Read the model definition and answer for the solid it produces. Units are mm, in the model's axes. A direction names the side the tool comes from. Round coordinates to 2 decimals unless told otherwise and drop trailing zeros. Order: outer loops, then holes, each group sorted by start corner. A loop starts at its lowest first (then second) coordinate and runs counter-clockwise, first axis right, second up.
from build123d import *

# Parameters (mm, degrees)
BENCH_FOOTPRINT_140X120_PROFILE_W       = 140
BENCH_FOOTPRINT_140X120_PROFILE_H       = 120
BENCH_FOOTPRINT_140X120_DEPTH           = 5
BACKBONE_START                          = -20
BACKBONE_PROFILE_W                      = 14
BACKBONE_PROFILE_H                      = 63
BACKBONE_DEPTH                          = 40
REMOVABLE_SERVO_MOUNT_M3_START          = -40
REMOVABLE_SERVO_MOUNT_M3_PROFILE_R      = 1.6
REMOVABLE_SERVO_MOUNT_M3_DEPTH          = 155.560027933
BEARING_BRIDGE_START                    = 39
BEARING_BRIDGE_PROFILE_W                = 53
BEARING_BRIDGE_PROFILE_H                = 40
BEARING_BRIDGE_DEPTH                    = 4
BRIDGE_HORN_CLEARANCE_START             = 38
BRIDGE_HORN_CLEARANCE_PROFILE_R         = 14
BRIDGE_HORN_CLEARANCE_DEPTH             = 77.560027933
DRIVE_COLLAR_CHAMBER_START              = 43
DRIVE_COLLAR_CHAMBER_PROFILE_R          = 18
DRIVE_COLLAR_CHAMBER_PROFILE_R_2        = 14
DRIVE_COLLAR_CHAMBER_DEPTH              = 5
BEARING_TOWER_START                     = 48
BEARING_TOWER_PROFILE_R                 = 18
BEARING_TOWER_PROFILE_R_2               = 11.1
BEARING_TOWER_DEPTH                     = 23
BEARING_SEPARATION_SHOULDER_START       = 55
BEARING_SEPARATION_SHOULDER_PROFILE_R   = 11.1
BEARING_SEPARATION_SHOULDER_PROFILE_R_2 = 9
BEARING_SEPARATION_SHOULDER_DEPTH       = 8
BENCH_CLAMP_HOLES_START                 = -1
BENCH_CLAMP_HOLES_PROFILE_R             = 2.75
BENCH_CLAMP_HOLES_DEPTH                 = 118.365802537
YAW_CROSSBOLT_ACCESS_START              = -40
YAW_CROSSBOLT_ACCESS_PROFILE_R          = 2.5
YAW_CROSSBOLT_ACCESS_DEPTH              = 157.365802537


with BuildPart() as part:
    # Bench_footprint_140x120_profile → Bench_footprint_140x120 (new body)
    with BuildSketch(Plane(origin=(0, 0, 0), x_dir=(1, 0, 0), z_dir=(0, 1, 0))):
        Rectangle(BENCH_FOOTPRINT_140X120_PROFILE_W, BENCH_FOOTPRINT_140X120_PROFILE_H)
    extrude(amount=BENCH_FOOTPRINT_140X120_DEPTH)

    # Backbone_profile → Backbone (add)
    with BuildSketch(Plane.XY.offset(BACKBONE_START)):
        with Locations((-28, 36.5)):
            Rectangle(BACKBONE_PROFILE_W, BACKBONE_PROFILE_H)
    extrude(amount=BACKBONE_DEPTH)

    # Removable_servo_mount_M3_profile → Removable_servo_mount_M3 (cut, through all)
    with BuildSketch(Plane(origin=(0, 0, 0), x_dir=(0, 0, -1), z_dir=(1, 0, 0)).offset(REMOVABLE_SERVO_MOUNT_M3_START)):
        with Locations(Location((12, 28, 0), (0, 0, 180))):
            Circle(REMOVABLE_SERVO_MOUNT_M3_PROFILE_R)
        with Locations(Location((-12, 28, 0), (0, 0, 180))):
            Circle(REMOVABLE_SERVO_MOUNT_M3_PROFILE_R)
    extrude(amount=REMOVABLE_SERVO_MOUNT_M3_DEPTH, mode=Mode.SUBTRACT)

    # Bearing_bridge_profile → Bearing_bridge (add)
    with BuildSketch(Plane(origin=(0, 0, 0), x_dir=(1, 0, 0), z_dir=(0, 1, 0)).offset(BEARING_BRIDGE_START)):
        with Locations((-8.5, 0)):
            Rectangle(BEARING_BRIDGE_PROFILE_W, BEARING_BRIDGE_PROFILE_H)
    extrude(amount=BEARING_BRIDGE_DEPTH)

    # Bridge_horn_clearance_profile → Bridge_horn_clearance (cut, through all)
    with BuildSketch(Plane(origin=(0, 0, 0), x_dir=(1, 0, 0), z_dir=(0, 1, 0)).offset(BRIDGE_HORN_CLEARANCE_START)):
        with Locations(Location((0, 0, 0), (0, 0, 90))):
            Circle(BRIDGE_HORN_CLEARANCE_PROFILE_R)
    extrude(amount=BRIDGE_HORN_CLEARANCE_DEPTH, mode=Mode.SUBTRACT)

    # Drive_collar_chamber_profile → Drive_collar_chamber (add)
    with BuildSketch(Plane(origin=(0, 0, 0), x_dir=(1, 0, 0), z_dir=(0, 1, 0)).offset(DRIVE_COLLAR_CHAMBER_START)):
        Circle(DRIVE_COLLAR_CHAMBER_PROFILE_R)
        with Locations(Location((0, 0, 0), (0, 0, 90))):
            Circle(DRIVE_COLLAR_CHAMBER_PROFILE_R_2, mode=Mode.SUBTRACT)
    extrude(amount=DRIVE_COLLAR_CHAMBER_DEPTH)

    # Bearing_tower_profile → Bearing_tower (add)
    with BuildSketch(Plane(origin=(0, 0, 0), x_dir=(1, 0, 0), z_dir=(0, 1, 0)).offset(BEARING_TOWER_START)):
        Circle(BEARING_TOWER_PROFILE_R)
        with Locations(Location((0, 0, 0), (0, 0, 270))):
            Circle(BEARING_TOWER_PROFILE_R_2, mode=Mode.SUBTRACT)
    extrude(amount=BEARING_TOWER_DEPTH)

    # Bearing_separation_shoulder_profile → Bearing_separation_shoulder (add)
    with BuildSketch(Plane(origin=(0, 0, 0), x_dir=(1, 0, 0), z_dir=(0, 1, 0)).offset(BEARING_SEPARATION_SHOULDER_START)):
        with Locations(Location((0, 0, 0), (0, 0, 270))):
            Circle(BEARING_SEPARATION_SHOULDER_PROFILE_R)
        with Locations(Location((0, 0, 0), (0, 0, 270))):
            Circle(BEARING_SEPARATION_SHOULDER_PROFILE_R_2, mode=Mode.SUBTRACT)
    extrude(amount=BEARING_SEPARATION_SHOULDER_DEPTH)

    # Bench_clamp_holes_profile → Bench_clamp_holes (cut, through all)
    with BuildSketch(Plane(origin=(0, 0, 0), x_dir=(1, 0, 0), z_dir=(0, 1, 0)).offset(BENCH_CLAMP_HOLES_START)):
        with Locations(Location((-55, -45, 0), (0, 0, 90))):
            Circle(BENCH_CLAMP_HOLES_PROFILE_R)
        with Locations(Location((55, -45, 0), (0, 0, 90))):
            Circle(BENCH_CLAMP_HOLES_PROFILE_R)
        with Locations(Location((-55, 45, 0), (0, 0, 90))):
            Circle(BENCH_CLAMP_HOLES_PROFILE_R)
        with Locations(Location((55, 45, 0), (0, 0, 90))):
            Circle(BENCH_CLAMP_HOLES_PROFILE_R)
    extrude(amount=BENCH_CLAMP_HOLES_DEPTH, mode=Mode.SUBTRACT)

    # Yaw_crossbolt_access_profile → Yaw_crossbolt_access (cut, through all)
    with BuildSketch(Plane(origin=(0, 0, 0), x_dir=(0, 0, -1), z_dir=(1, 0, 0)).offset(YAW_CROSSBOLT_ACCESS_START)):
        with Locations(Location((0, 45.5, 0), (0, 0, 90))):
            Circle(YAW_CROSSBOLT_ACCESS_PROFILE_R)
    extrude(amount=YAW_CROSSBOLT_ACCESS_DEPTH, mode=Mode.SUBTRACT)


solid = part.part
Q1. Straight lines are drawn through the part: probe 1 along X at (y, z) = (4, 45); probe 2 along X at (y, z) = (52, 0); probe 3 along Y at (x, z) = (-31.75, 12). For each, find the intervals that lie inside material, in ascending order.
Outcome:
probe 1: x = -70 to -57.75, -52.25 to 52.25, 57.75 to 70
probe 2: x = -35 to -21, -18 to -11.1, 11.1 to 18
probe 3: y = 0 to 26.4, 29.6 to 68
Q2. For faces 5 (the face through (18, 41, 0)), 6 (the face through (2.703, 58.944, 8.584)), 7 (the face through (-28, 68, 0)), 8 (the face through (-26, 37, 20)), determine the directions among +Z, -Z, +X, -X, +Y, -Y from which every point of the face is accessible in a straight line to the end or side of a thin tool.
Outcome:
face 5: +Z, -Z, +X, +Y
face 6: +Y
face 7: +Z, -Z, -X, +Y
face 8: +Z, +X, -X, +Y
Q3. A cutting plane is placed at C-C, the plane x = 0. Give the vertices of the cut face in (y, z).
Outcome:
outline: (0, -60) - (5, -60) - (5, 60) - (0, 60) - close; (39, -20) - (43, -20) - (43, -18) - (71, -18) - (71, -11.1) - (63, -11.1) - (63, -9) - (55, -9) - (55, -11.1) - (48, -11.1) - (48, -14) - (39, -14) - close; (39, 14) - (48, 14) - (48, 11.1) - (55, 11.1) - (55, 9) - (63, 9) - (63, 11.1) - (71, 11.1) - (71, 18) - (43, 18) - (43, 20) - (39, 20) - close
Q4. A cutting plane is placed at B-B, the plane y = 28. Give the vertices of the cut face in (x, z).
Outcome:
outline: (-35, -20) - (-21, -20) - (-21, -13.6) - (-35, -13.6) - close; (-35, -10.4) - (-21, -10.4) - (-21, 10.4) - (-35, 10.4) - close; (-35, 13.6) - (-21, 13.6) - (-21, 20) - (-35, 20) - close
Q5. Flat-ended cylindrical pins translate along their axes: pin 1 (7 mm diameter, centred on x = -55, z = 45, fed in from -Y); pin 2 (3 mm diameter, centred on y = 28, z = 12, fed in from -X); pin 3 (4 mm diameter, centred on x = -16.5, y = 62.5, fed in from -Z); pin 4 (1 mm diameter, centred on x = -42, z = -32, fed in from +Y). Find the tip coordinate at first contact, or state that the pin passes through.
Outcome:
pin 1: stops at y = 0
pin 2: passes through
pin 3: stops at z = -10.67
pin 4: stops at y = 5
Q6. A cutting plane is placed at A-A, the plane z = -45. Give the vertices of the cut face in (x, y), plus the area to 3 significant figures.
Outcome:
outline: (-70, 0) - (-57.75, 0) - (-57.75, 5) - (-70, 5) - close; (-52.25, 0) - (52.25, 0) - (52.25, 5) - (-52.25, 5) - close; (57.75, 0) - (70, 0) - (70, 5) - (57.75, 5) - close
area: 645 mm2
Q7. For a pull along X with two mould halves and no side action, classify faces 1 (the face through (70, 2, 1)), 2 (the face through (53.141, 2.465, 47.027)), 3 (the face through (9, 55, -2)), 4 (the face through (-1, 0, -1)) as released by +X, released by -X, zero draft, split by the parting line, or undercut.
Outcome:
face 1: released by +X
face 2: undercut
face 3: undercut
face 4: zero draft
Q8. A cutting plane is placed at D-D, the plane y = 10. Give the vertices of the cut face in (x, z), plus the area to 3 significant figures.
Outcome:
outline: (-35, -20) - (-21, -20) - (-21, 20) - (-35, 20) - close
area: 560 mm2
